```python
from build123d import *

# Parameters (mm, degrees)
SKETCH3_R           = 63.5
SKETCH5_R           = 38.1
SKETCH6_W           = 152.4
SKETCH6_H           = 152.4
BOSS_EXTRUDE1_DEPTH = 25.4
SKETCH7_R           = 6.35
BOSS_EXTRUDE2_DEPTH = 25.4


with BuildPart() as part:
    # Sketch3 → Loft1 section 0
    with BuildSketch(Plane(origin=(0, 0, 0), x_dir=(1, 0, 0), z_dir=(0, 1, 0))):
        Circle(SKETCH3_R)
    # Sketch5 → Loft1 section 1
    with BuildSketch(Plane(origin=(0, 50.8, 0), x_dir=(1, 0, 0), z_dir=(0, 1, 0))):
        Circle(SKETCH5_R)
    loft()

    # Sketch6 → Boss-Extrude1 (add)
    with BuildSketch(Plane.XZ):
        Rectangle(SKETCH6_W, SKETCH6_H)
    extrude(amount=BOSS_EXTRUDE1_DEPTH)

    # Sketch7 → Boss-Extrude2 (add)
    with BuildSketch(Plane(origin=(0, 50.8, 0), x_dir=(1, 0, 0), z_dir=(0, 1, 0))):
        with Locations(Location((0, 0, 0), (0, 0, 270))):
            Circle(SKETCH7_R)
    extrude(amount=BOSS_EXTRUDE2_DEPTH)


solid = part.part
```
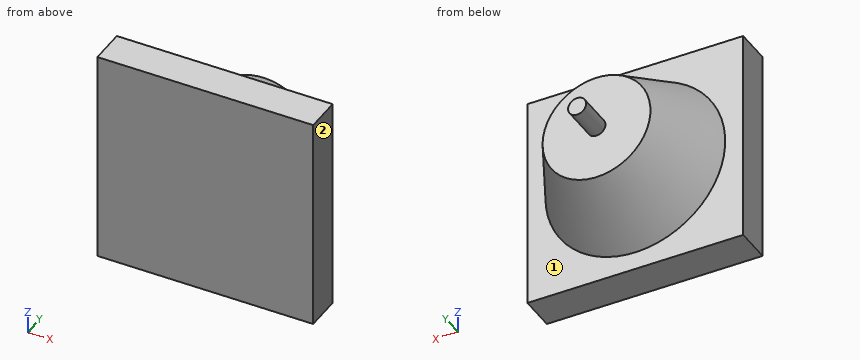
Geometry: final body of the model. Coordinates: model frame, mm. Face numbers are marked on the shaded views. A direction names the side the tool comes from. Round coordinates to 2 decimals unless told otherwise and drop trailing zeros. Loops run counter-clockwise (first coordinate to the right, second up) from the corner with the lowest first, then second, coordinate; pieces in that order, holes last. Notation, with made-up numbers: (68, 88.5) -> (89, 88.5) arc R25 ccw to (89, 111.5) -> close; hole circle Ø9 at (82, 2). An arc over 180 degrees is marked (long way). Use one line per item in the form item = value. Start each with the question number.
1) Section A-A on x = 0. Output: boundary loops of the cut face in (y, z), then the cut area to 3 significant figures.
2) Section C-C on z = 66.5. Output: boundary loops of the cut face in (x, y), then the cut area to 3 significant figures.
3) Line query: L1, parallel to Y at x = 36, z = 69.5; L2, parallel to Y at x = -21.5, z = 11; L3, parallel to Z at x = -39, y = 0.5. Output: solid intervals per line, ascending.
4) Section B-B on y = 13. Output: boundary loops of the cut face in (x, z).
5) Section D-D on y = 24. Output: boundary loops of the cut face in (x, z), then the cut area to 3 significant figures.
6) Access query for the marked faces 1 and 2. Directions: +Z, -Z, +X, -X, +Y, -Y. A direction counts if a zero-diameter tool reaches every point of the face in a straight line with its end or side. Return the directions, or none.
7) First-contact query: P1, Ø6, axis at y = 32, z = 34, coming from the -X side. Flat tip, straight axial feed; report the tip coordinate or a pass-through.
Response:
q1.outline = (-25.4, -76.2) -> (0, -76.2) -> (0, -63.5) -> (50.8, -38.1) -> (50.8, -6.35) -> (76.2, -6.35) -> (76.2, 6.35) -> (50.8, 6.35) -> (50.8, 38.1) -> (0, 63.5) -> (0, 76.2) -> (-25.4, 76.2) -> close
q1.area = 9,350 mm^2
q2.outline = (-76.2, -25.4) -> (76.2, -25.4) -> (76.2, 0) -> (-76.2, 0) -> close
q2.area = 3,870 mm^2
q3.L1 = -25.4 to 0
q3.L2 = -25.4 to 50.8
q3.L3 = -49.8 to 49.8
q4.outline = circle Ø114 at (0, 0)
q5.outline = circle Ø103 at (0, 0)
q5.area = 8,330 mm^2
q6.face_1 = +Y
q6.face_2 = +Z, -Z, +X, +Y, -Y
q7.P1 = -36.66
